Can you work these out from the model? Positions are in its coordinate system, mm. A direction names the side the tool comes from. Give positions to 0.01 mm unless a question says otherwise; leave off trailing zeros. Loops run counter-clockwise (first coordinate to the right, second up) from the corner with the lowest first, then second, coordinate; pieces in that order, holes last. Notation, with made-up numbers: (19.25, -35.5) - (48.25, -35.5) arc R12 cw to (48.25, -23.5) - close; hole circle Ø6 at (-26, -7). An arc over 180 degrees is marked (long way). Use a Markdown table: item, result. Add a question column.
```python
from build123d import *

# Parameters (mm, degrees)
SKETCH1_R           = 3.175
BOSS_EXTRUDE1_DEPTH = 6.35
SKETCH2_R           = 5.08
BOSS_EXTRUDE2_DEPTH = 2.54
SKETCH3_R           = 3.81
BOSS_EXTRUDE3_DEPTH = 19.05
SKETCH4_R           = 5.08
BOSS_EXTRUDE4_DEPTH = 2.54
SKETCH5_R           = 3.175
BOSS_EXTRUDE5_DEPTH = 6.35


with BuildPart() as part:
    # Sketch1 → Boss-Extrude1 (new body)
    with BuildSketch(Plane.XY):
        Circle(SKETCH1_R)
    extrude(amount=BOSS_EXTRUDE1_DEPTH)

    # Sketch2 → Boss-Extrude2 (add)
    with BuildSketch(Plane.XY.offset(6.35)):
        Circle(SKETCH2_R)
    extrude(amount=BOSS_EXTRUDE2_DEPTH)

    # Sketch3 → Boss-Extrude3 (add)
    with BuildSketch(Plane.XY.offset(8.89)):
        with Locations(Location((0, 0, 0), (0, 0, 180))):
            Circle(SKETCH3_R)
    extrude(amount=BOSS_EXTRUDE3_DEPTH)

    # Sketch4 → Boss-Extrude4 (add)
    with BuildSketch(Plane.XY.offset(27.94)):
        Circle(SKETCH4_R)
    extrude(amount=BOSS_EXTRUDE4_DEPTH)

    # Sketch5 → Boss-Extrude5 (add)
    with BuildSketch(Plane.XY.offset(30.48)):
        Circle(SKETCH5_R)
    extrude(amount=BOSS_EXTRUDE5_DEPTH)


solid = part.part
```
1. Will these pins go through, and if not, where does the flat tip stop? P1, Ø5, axis at x = -1.5, y = -0.5, coming from the -Z side; P2, Ø1, axis at x = -3.5, z = 23.5, coming from the -Y side; P3, Ø6, axis at y = -1, z = 17.5, coming from the -X side; P4, Ø4, axis at x = -2.5, z = 24, coming from the +Y side.
2. If we mould it in two halves opening along Z, with no side actions, what happens to faces 1 (the face through (0.496, -3.778, 18.282)), 2 (the face through (-0.69, -3.1, 3.13)), 3 (the face through (0, 0, 0)), 4 (the face through (0, 0, 36.83))? For each: released by +Z, released by -Z, zero draft, split by the parting line, or undercut.
3. On a 3-axis mill with a long thin cutter (end or side, diameter ignored), from which of +Z, -Z, +X, -X, +Y, -Y can I reach the whole of each face in a straight line? I mean faces 5 (the face through (1, 4, 8.89)), 6 (the face through (3.3, -1.1, 6.35)), 7 (the face through (-0.661, 5.037, 29.192)), 8 (the face through (-0.69, -3.1, 33.61)). Say none if no direction works.
4. Suppose I cut it at A-A (x = 0). List the corners of the cut face in (y, z) for me (3 decimals).
5. Suppose I cut it at B-B (x = -4.25). List the corners of the cut face in (y, z) for me.
6. Please list where these lines run through material, in increasing order: line 1 along Z through (x, y) = (2, 2.75); line 2 along Z through (x, y) = (-4, 2.25); line 3 along X through (y, z) = (2.5, 10.5). Write a range as [from, to].
7. Suppose I cut it at C-C (y = 1). List the corners of the cut face in (x, z) for me.
8. Suppose I cut it at D-D (z = 18). List the corners of the cut face in (x, y) for me.
Results below:
| question | item | result |
|---|---|---|
| 1 | P1 | z = 0 |
| 1 | P2 | y = -2.35 |
| 1 | P3 | x = -3.81 |
| 1 | P4 | y = 3.78 |
| 2 | face 1 | undercut |
| 2 | face 2 | zero draft |
| 2 | face 3 | released by -Z |
| 2 | face 4 | released by +Z |
| 3 | face 5 | none |
| 3 | face 6 | -Z |
| 3 | face 7 | +Z, -Z |
| 3 | face 8 | +Z |
| 4 | outline | (-5.08, 6.35) - (-3.175, 6.35) - (-3.175, 0) - (3.175, 0) - (3.175, 6.35) - (5.08, 6.35) - (5.08, 8.89) - (3.81, 8.89) - (3.81, 27.94) - (5.08, 27.94) - (5.08, 30.48) - (3.175, 30.48) - (3.175, 36.83) - (-3.175, 36.83) - (-3.175, 30.48) - (-5.08, 30.48) - (-5.08, 27.94) - (-3.81, 27.94) - (-3.81, 8.89) - (-5.08, 8.89) - close |
| 5 | outline | (-2.78, 6.35) - (2.78, 6.35) - (2.78, 8.89) - (-2.78, 8.89) - close; (-2.78, 27.94) - (2.78, 27.94) - (2.78, 30.48) - (-2.78, 30.48) - close |
| 6 | line 1 | [6.35, 30.48] |
| 6 | line 2 | [6.35, 8.89], [27.94, 30.48] |
| 6 | line 3 | [-2.88, 2.88] |
| 7 | outline | (-4.98, 6.35) - (-3.01, 6.35) - (-3.01, 0) - (3.01, 0) - (3.01, 6.35) - (4.98, 6.35) - (4.98, 8.89) - (3.68, 8.89) - (3.68, 27.94) - (4.98, 27.94) - (4.98, 30.48) - (3.01, 30.48) - (3.01, 36.83) - (-3.01, 36.83) - (-3.01, 30.48) - (-4.98, 30.48) - (-4.98, 27.94) - (-3.68, 27.94) - (-3.68, 8.89) - (-4.98, 8.89) - close |
| 8 | outline | circle Ø7.62 at (0, 0) |
